Geometry: final body of the model. Coordinates: model frame, mm. Face numbers are marked on the shaded views. A direction names the side the tool comes from. Round coordinates to 2 decimals unless told otherwise and drop trailing zeros. Order: outer loops, then holes, each group sorted by start corner. A loop starts at its lowest first (then second) coordinate and runs counter-clockwise, first axis right, second up. Notation, with made-up numbers: M 11,15.5 L 16,15.5 A8 ccw 16,29.5 Z; hole C 27,-18.75 d8. An arc over 180 degrees is marked long. Return JSON: item names as keys, results as strings. Group by question number.
Q1. Contact query for flat-ended pins moving along their axis: pin 1 (10.5 mm diameter, centred on y = 0, z = 0, fed in from -X); pin 2 (9 mm diameter, centred on x = -77.5, y = 0, fed in from +Z); pin 3 (3 mm diameter, centred on x = -25, z = -18.5, fed in from -Y). Output: stop coordinate, or through.
Q2. Cut plane B-B on x = -29. Output: boundary loops of the cut face in (y, z), and give its area (3 significant figures).
Q3. Ray query, probe 1 along Y at (x, z) = (-71.5, 0); probe 2 along X at (y, z) = (0, -9); probe 3 along X at (y, z) = (14, -22.5). Return the intervals inside material, ascending.
Q4. Access query for the marked faces 1 and 2. Directions: +Z, -Z, +X, -X, +Y, -Y. A direction counts if a zero-diameter tool reaches every point of the face in a straight line with its end or side. Return the directions, or none.
Q5. Mould query, pull axis Y, two halves, no side actions, for the marked faces 3, 4 and 5. Classes: released by +Y, released by -Y, zero draft, split by the parting line, or undercut.
Q6. Cut plane A-A on x = -94. Output: boundary loops of the cut face in (y, z).
```python
from build123d import *

# Parameters (mm, degrees)
SKETCH_2_R                = 4
CUT_EXTRUDE_1_DEPTH       = 30
CHAMFER_1_SIZE            = 2
CHAMFER_2_SIZE            = 3
CHAMFER_2_SIZE2           = 0.803847577
SKETCH_6_R                = 15
CUT_EXTRUDE_3_DEPTH       = 10
HOLE_WIZARD_8_0_8_1_D     = 8
HOLE_WIZARD_8_0_8_1_DEPTH = 80
HOLE_WIZARD_8_0_8_1_TIP   = 2.403442476
M10X1_0_1_D               = 9
M10X1_0_1_DEPTH           = 15
M10X1_0_1_TIP             = 2.703872786


with BuildPart() as part:
    # 草图1 → 旋转1 (revolve)
    with BuildSketch(Plane.XY, mode=Mode.PRIVATE) as revolve_1_sk:
        with BuildLine():
            Line((0, 0), (0, 27.5))
            Line((0, 27.5), (-71.5, 27.5))
            ThreePointArc((-71.5, 27.5), (-77.5, 25.5), (-83.5, 27.5))
            Line((-83.5, 27.5), (-149, 27.5))
            Line((-149, 27.5), (-149, 22.5))
            Line((-149, 22.5), (-160, 22.5))
            Line((-160, 22.5), (-160, 0))
            Line((-160, 0), (0, 0))
        make_face()
    revolve(revolve_1_sk.sketch.rotate(Axis((0, 0, 0), (-1, 0, 0)), 90), axis=Axis((0, 0, 0), (-1, 0, 0)))

    # 草图2 → 切除-拉伸1 (cut, symmetric)
    with BuildSketch(Plane.XY):
        with Locations((-77.5, 0)):
            Circle(SKETCH_2_R)
    extrude(amount=CUT_EXTRUDE_1_DEPTH, both=True, mode=Mode.SUBTRACT)

    # 倒角1
    chamfer_1_edges = [part.edges().sort_by_distance(p)[0] for p in [
        (-160, 0, 22.5),
    ]]
    chamfer(chamfer_1_edges, length=CHAMFER_1_SIZE)

    # 倒角2
    chamfer_2_edges = [part.edges().sort_by_distance(p)[0] for p in [
        (0, 0, 27.5),
    ]]
    chamfer_2_side = [part.faces().sort_by_distance(p)[0] for p in [
        (-35.75, 0, 27.5),
    ]]
    chamfer(chamfer_2_edges, length=CHAMFER_2_SIZE, length2=CHAMFER_2_SIZE2, reference=chamfer_2_side[0])

    # 草图6 → 切除-拉伸3 (cut)
    with BuildSketch(Plane.ZY.offset(160)):
        Circle(SKETCH_6_R)
    extrude(amount=-CUT_EXTRUDE_3_DEPTH, mode=Mode.SUBTRACT)

    # Ø8.0 (8) 直径孔1
    with Locations(Plane(origin=(-150, 0, 0), x_dir=(0, 0, -1), z_dir=(-1, 0, 0))):
        with Locations((0, 0)):
            Hole(HOLE_WIZARD_8_0_8_1_D / 2, depth=HOLE_WIZARD_8_0_8_1_DEPTH)
            with Locations((0, 0, -(HOLE_WIZARD_8_0_8_1_DEPTH + HOLE_WIZARD_8_0_8_1_TIP / 2))):  # 118° drill point
                Cone(0, HOLE_WIZARD_8_0_8_1_D / 2, HOLE_WIZARD_8_0_8_1_TIP, mode=Mode.SUBTRACT)

    # M10x1.0 螺纹孔1
    with Locations(Plane.ZY.offset(150)):
        with Locations((0, 0)):
            Hole(M10X1_0_1_D / 2, depth=M10X1_0_1_DEPTH)
            with Locations((0, 0, -(M10X1_0_1_DEPTH + M10X1_0_1_TIP / 2))):  # 118° drill point
                Cone(0, M10X1_0_1_D / 2, M10X1_0_1_TIP, mode=Mode.SUBTRACT)


solid = part.part
```
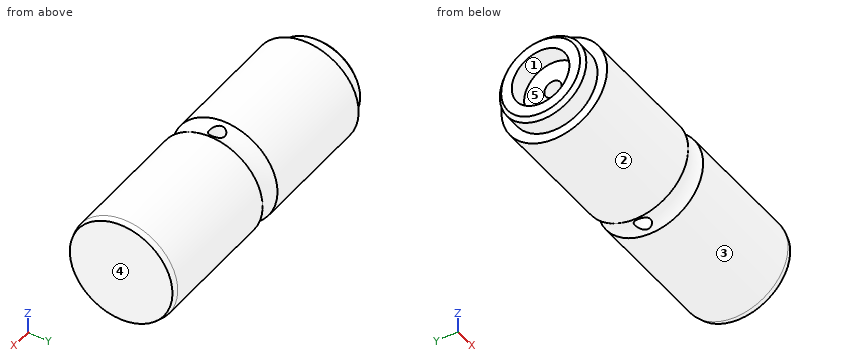
Result sheet:
{
 "1": {"pin 1": "stops at x = -150", "pin 2": "stops at z = 26.57", "pin 3": "stops at y = -21.62"},
 "2": {"outline": "C 0,0 d55", "area": "2,380 mm²"},
 "3": {"probe 1": "y = -27.5 to -4, 4 to 27.5", "probe 2": "x = -150 to -81.5, -73.5 to 0", "probe 3": "x = -149 to -81.86, -73.14 to 0"},
 "4": {"face 1": "-X", "face 2": "+X, -X"},
 "5": {"face 3": "split by the parting line", "face 4": "zero draft", "face 5": "undercut"},
 "6": {"outline": "C 0,0 d55; hole C 0,0 d8"}
}
